Input: part model. Units: mm. Frame: model coordinates. Face numbers are marked on the shaded views. Give positions to 0.01 mm unless a question says otherwise; leave off trailing zeros. Loops run counter-clockwise (first coordinate to the right, second up) from the corner with the lowest first, then second, coordinate; pieces in that order, holes last. Notation, with made-up numbers: M 74,5.5 L 116,5.5 A19 ccw 116,32.5 Z; hole C -27.75,-8.5 d7. An arc over 180 degrees is marked long. Use a Markdown table: item, result. Add a question column.
from build123d import *

# Parameters (mm, degrees)
SKETCH1_W                       = 40
SKETCH1_H                       = 6
BOSS_EXTRUDE1_DEPTH             = 5
CBORE_FOR_M3_SBHCS1_D           = 3.4
CBORE_FOR_M3_SBHCS1_DEPTH       = 7.5
CBORE_FOR_M3_SBHCS1_CBORE_D     = 5.9
CBORE_FOR_M3_SBHCS1_CBORE_DEPTH = 1.65
CBORE_FOR_M3_SBHCS1_TIP         = 1.021463052


with BuildPart() as part:
    # Sketch1 → Boss-Extrude1 (new body)
    with BuildSketch(Plane(origin=(0, 0, 0), x_dir=(1, 0, 0), z_dir=(0, 1, 0))):
        with Locations((20, 3)):
            Rectangle(SKETCH1_W, SKETCH1_H)
    extrude(amount=BOSS_EXTRUDE1_DEPTH)

    # CBORE for M3 SBHCS1
    with Locations(Plane(origin=(0, 5, 0), x_dir=(1, 0, 0), z_dir=(0, 1, 0))):
        with Locations((37, 3), (19, 3)):
            CounterBoreHole(CBORE_FOR_M3_SBHCS1_D / 2, CBORE_FOR_M3_SBHCS1_CBORE_D / 2, CBORE_FOR_M3_SBHCS1_CBORE_DEPTH, depth=CBORE_FOR_M3_SBHCS1_DEPTH)
            with Locations((0, 0, -(CBORE_FOR_M3_SBHCS1_DEPTH + CBORE_FOR_M3_SBHCS1_TIP / 2))):  # 118° drill point
                Cone(0, CBORE_FOR_M3_SBHCS1_D / 2, CBORE_FOR_M3_SBHCS1_TIP, mode=Mode.SUBTRACT)


solid = part.part
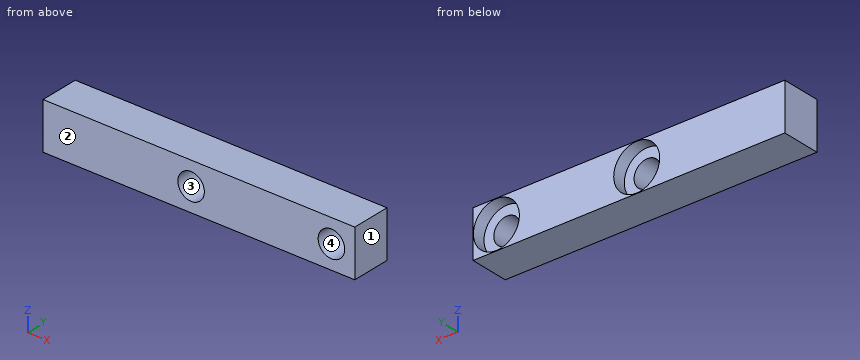
1) Contact query for a flat-ended pin moving along its axis: P1, Ø2.5, axis at x = 37, z = -3, coming from the +Y side. Output: stop coordinate, or through.
2) Section query B-B, the plane z = -2.45. Return the cut outline in (x, y).
3) Pull-direction query (X, two-part tool) for the marked faces 1, 2, 3 and 4; classes: pulls with the +X half, pulls with the -X half, needs draft (parallel to the pull), parting line crosses it, or undercut.
4) Section query C-C, the plane y = 3.8. Return the cut outline in (x, z).
5) Section query A-A, the plane x = 19. Return the cut outline in (y, z).
6) Section query D-D, the plane z = -0.8. Return the cut outline in (x, y).
7) Ray query, line 1 (X direction, y = 3.2, z = -3.15); line 2 (X direction, y = 2.1, z = -2.3); line 3 (Z direction, x = 19, y = 2.15). Return the intervals inside material, ascending. Write a range as [from, to].
Entries:
| question | item | result |
|---|---|---|
| 1 | P1 | passes through |
| 2 | outline | M 0,0 L 17.39,0 L 17.39,3.35 L 16.1,3.35 L 16.1,5 L 0,5 Z; M 20.61,0 L 35.39,0 L 35.39,3.35 L 34.1,3.35 L 34.1,5 L 21.9,5 L 21.9,3.35 L 20.61,3.35 Z; M 38.61,0 L 40,0 L 40,5 L 39.9,5 L 39.9,3.35 L 38.61,3.35 Z |
| 3 | face 1 | pulls with the +X half |
| 3 | face 2 | needs draft |
| 3 | face 3 | undercut |
| 3 | face 4 | undercut |
| 4 | outline | M 0,-6 L 40,-6 L 40,0 L 0,0 Z; hole C 19,-3 d5.9; hole C 37,-3 d5.9 |
| 5 | outline | M 0,-6 L 5,-6 L 5,-5.95 L 3.35,-5.95 L 3.35,-4.7 L 0,-4.7 Z; M 0,-1.3 L 3.35,-1.3 L 3.35,-0.05 L 5,-0.05 L 5,0 L 0,0 Z |
| 6 | outline | M 0,0 L 40,0 L 40,5 L 38.97,5 L 38.97,3.35 L 35.03,3.35 L 35.03,5 L 20.97,5 L 20.97,3.35 L 17.03,3.35 L 17.03,5 L 0,5 Z |
| 7 | line 1 | x = [0, 17.31], [20.69, 35.31], [38.69, 40] |
| 7 | line 2 | x = [0, 17.45], [20.55, 35.45], [38.55, 40] |
| 7 | line 3 | z = [-6, -4.7], [-1.3, 0] |
